```python
from build123d import *

# Parameters (mm, degrees)
F0_R      = 15.875
F1_DEPTH  = 12.7
F5_R      = 3.175
F6_DEPTH  = 12.701
F7_R      = 20.024716
F7_R_2    = 12.065
F8_DEPTH  = 12.701
F10_R     = 20.449892
F10_R_2   = 1.769063
F11_DEPTH = 6.35


with BuildPart() as f1:
    # F0 (on Top) → F1 (new body)
    with BuildSketch(Plane.XY):
        Circle(F0_R)
    extrude(amount=F1_DEPTH)

    # F2 (on Right) → F4 (revolve, cut)
    with BuildSketch(Plane.YZ):
        with BuildLine():
            Line((-12.065, 8.466667), (-12.065, 4.233333))
            Line((-12.065, 4.233333), (-9.948333, 4.233333))
            ThreePointArc((-9.948333, 4.233333), (-7.831667, 6.35), (-9.948333, 8.466667))
            Line((-9.948333, 8.466667), (-12.065, 8.466667))
        make_face()
    revolve(axis=Axis((0, 0, 11.412669), (0, 0, 1)), mode=Mode.SUBTRACT)

    # F5 (on face) → F6 (cut, through all)
    with BuildSketch(Plane.XY.offset(12.7)):
        Circle(F5_R)
    extrude(amount=-F6_DEPTH, mode=Mode.SUBTRACT)

    # F7 (on face) → F8 (cut, through all)
    with BuildSketch(Plane.XY.offset(12.7)):
        Circle(F7_R)
        Circle(F7_R_2, mode=Mode.SUBTRACT)
    extrude(amount=-F8_DEPTH, mode=Mode.SUBTRACT)

    # F10 (on face) → F11 (cut, through all)
    with BuildSketch(Plane.XY.offset(12.7)):
        Circle(F10_R)
        Circle(F10_R_2, mode=Mode.SUBTRACT)
    extrude(amount=-F11_DEPTH, mode=Mode.SUBTRACT)


solid = f1.part
```
The model under review builds one solid part; all positions refer to its coordinate system, in mm. A direction names the side the tool comes from. Give positions to 0.01 mm unless a question says otherwise; leave off trailing zeros. Write each loop counter-clockwise with the first axis right and the second up, starting at its lowest first coordinate (ties: lowest second). Pieces come first, ordered by that corner, then holes. Notation, with made-up numbers: M -31,27 L -17,27 A27 cw -17,45 Z; hole C -8,76.5 d2. An arc over 180 degrees is marked long. Write item = value, one per line. Start each with the question number.
Q1. Machinability: for faces 1 (the face through (-0.1, -3.4, 6.35)), 2 (the face through (10, -2, 4.233)), which of the approach directions +Z, -Z, +X, -X, +Y, -Y give a long, thin tool a straight path to every point of the face, cutting with its end or side? Answer none if there is none.
Q2. We need section D-D (y = 10.5). State the section outline as (x, z) points.
Q3. For line 1 (Y direction, x = 0, z = 1.75) (3 decimals); line 2 (Z direction, x = -11, y = 0.25); line 3 (X direction, y = 0.5, z = 2.75), list the stretches that pass through material, from the lowest coordinate up.
Q4. We need section A-A (x = 0). State the section outline as (y, z) points (3 decimals), plus the area to 3 significant figures.
Q5. Mouldability with a two-part tool opening along X and no side actions: class faces 3 (the face through (-0.69, -3.1, 3.22)), 4 (the face through (3, -3, 0)), 5 (the face through (11.145, -4.621, 2.146)) as released by +X, released by -X, zero draft, split by the parting line, or undercut.
Q6. We need section C-C (z = 3). State the section outline as (x, y) points (3 decimals).
Result set:
q1.face_1 = +Z, +X, -X, +Y, -Y
q1.face_2 = +Z
q2.outline = M -5.94,0 L 5.94,0 L 5.94,4.23 L -5.94,4.23 Z
q3.line_1 = -12.065 to -3.175, 3.175 to 12.065
q3.line_2 = 0 to 4.23
q3.line_3 = -12.05 to -3.14, 3.14 to 12.05
q4.outline = M -12.065,0 L -3.175,0 L -3.175,6.35 L -7.832,6.35 A2.117 cw -9.948,4.233 L -12.065,4.233 Z; M 3.175,0 L 12.065,0 L 12.065,4.233 L 9.948,4.233 A2.117 cw 7.832,6.35 L 3.175,6.35 Z
q4.area = 96.9 mm2
q5.face_3 = undercut
q5.face_4 = zero draft
q5.face_5 = split by the parting line
q6.outline = C 0,0 d24.13; hole C 0,0 d6.35
